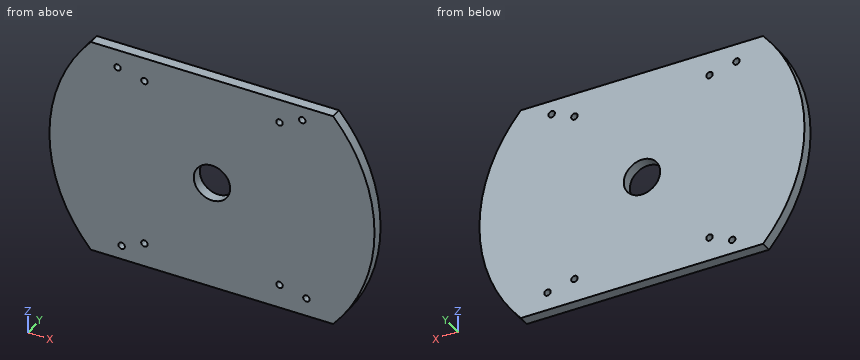
from build123d import *

# Parameters (mm, degrees)
SKETCH1_R           = 75
SKETCH1_R_2         = 1.5
SKETCH1_R_3         = 8.4
BOSS_EXTRUDE1_DEPTH = 5
CUT_EXTRUDE1_START  = -10
CUT_EXTRUDE1_DEPTH  = 10


with BuildPart() as part:
    # Sketch1 → Boss-Extrude1 (new body)
    with BuildSketch(Plane(origin=(0, 0, 0), x_dir=(1, 0, 0), z_dir=(0, 1, 0))):
        with Locations(Location((0, 0, 0), (0, 0, 270))):
            Circle(SKETCH1_R)
        with Locations(Location((-41.664692583, 43.590634223, 0), (0, 0, 270))):
            Circle(SKETCH1_R_2, mode=Mode.SUBTRACT)
        with Locations(Location((43.590634223, 41.664692583, 0), (0, 0, 270))):
            Circle(SKETCH1_R_2, mode=Mode.SUBTRACT)
        with Locations(Location((41.664692583, -43.590634223, 0), (0, 0, 270))):
            Circle(SKETCH1_R_2, mode=Mode.SUBTRACT)
        with Locations(Location((-43.590634223, -41.664692583, 0), (0, 0, 270))):
            Circle(SKETCH1_R_2, mode=Mode.SUBTRACT)
        with Locations(Location((-31.164692583, 39.090634223, 0), (0, 0, 270))):
            Circle(SKETCH1_R_2, mode=Mode.SUBTRACT)
        with Locations(Location((0, 0, 0), (0, 0, 270))):
            Circle(SKETCH1_R_3, mode=Mode.SUBTRACT)
        with Locations(Location((31.164692583, 39.090634223, 0), (0, 0, 270))):
            Circle(SKETCH1_R_2, mode=Mode.SUBTRACT)
        with Locations(Location((31.164692583, -39.090634223, 0), (0, 0, 270))):
            Circle(SKETCH1_R_2, mode=Mode.SUBTRACT)
        with Locations(Location((-31.164692583, -39.090634223, 0), (0, 0, 270))):
            Circle(SKETCH1_R_2, mode=Mode.SUBTRACT)
    extrude(amount=BOSS_EXTRUDE1_DEPTH)

    # Sketch3 → Cut-Extrude1 (cut)
    with BuildSketch(Plane(origin=(0, 5, 0), x_dir=(1, 0, 0), z_dir=(0, 1, 0)).offset(CUT_EXTRUDE1_START)):
        with BuildLine():
            Line((-55.901699437, 50), (0, 50))
            Line((0, 50), (55.901699437, 50))
            ThreePointArc((55.901699437, 50), (0, 75), (-55.901699437, 50))
        make_face()
        with BuildLine():
            Line((55.901699437, -50), (0, -50))
            Line((0, -50), (-55.901699437, -50))
            ThreePointArc((-55.901699437, -50), (0, -75), (55.901699437, -50))
        make_face()
    extrude(amount=CUT_EXTRUDE1_DEPTH, mode=Mode.SUBTRACT)


solid = part.part
The listing builds one solid part. Answer for the finished solid, in the listing's coordinates (mm). Give positions to 0.01 mm unless a question says otherwise; leave off trailing zeros. Loops run counter-clockwise (first coordinate to the right, second up) from the corner with the lowest first, then second, coordinate; pieces in that order, holes last. Notation, with made-up numbers: (33, 31.5) - (38, 31.5) arc R25 ccw to (38, 61.5) - close; hole circle Ø4 at (36, 89). An arc over 180 degrees is marked (long way). Answer as a JSON object with one key per item and string values.
1. A cutting plane is placed at D-D (x = 62). Write down the section's boundary in (y, z).
Determined:
{"outline": "(0, -42.2) - (5, -42.2) - (5, 42.2) - (0, 42.2) - close"}
2. A cutting plane is placed at B-B (x = 0). Write down the section's boundary in (y, z), then the cut area to 3 significant figures.
Determined:
{"outline": "(0, -50) - (5, -50) - (5, -8.4) - (0, -8.4) - close; (0, 8.4) - (5, 8.4) - (5, 50) - (0, 50) - close", "area": "416 mm²"}
3. A cutting plane is placed at C-C (y = 1.55). Give the number of separate pieces and of enclosed holes in the cut face, then the cut area to 3 significant figures.
Determined:
{"separate pieces": "1", "enclosed holes": "9", "area": "13,500 mm²"}
4. A cutting plane is placed at A-A (z = 0). Write down the section's boundary in (x, y), then the cut area to 3 significant figures.
Determined:
{"outline": "(-75, 0) - (-8.4, 0) - (-8.4, 5) - (-75, 5) - close; (8.4, 0) - (75, 0) - (75, 5) - (8.4, 5) - close", "area": "666 mm²"}
5. A flat-ended cylindrical pin translates along its axis: pin 1 Ø13.5 at (x, z) = (0, 0) entering from -Y. Find the tip coordinate at first contact, or state that the pin passes through.
Determined:
{"pin 1": "through"}
6. Find the intervals of material crossed by L1, parallel to X at y = 3.85, z = 0; L2, parallel to X at y = 3.95, z = -40; L3, parallel to X at y = 4.1, z = 4.5, in increasing order. Write a range as [from, to].
Determined:
{"L1": "[-75, -8.4], [8.4, 75]", "L2": "[-63.44, -32.36], [-29.97, 29.97], [32.36, 63.44]", "L3": "[-74.86, -7.09], [7.09, 74.86]"}
